For this review, take the finished solid that the model builds, in its own axes (mm). Round coordinates to 2 decimals unless told otherwise and drop trailing zeros. Write each loop counter-clockwise with the first axis right and the second up, starting at its lowest first coordinate (ties: lowest second). Pieces come first, ordered by that corner, then holes. Notation, with made-up numbers: (-4.75, -26.5) - (47.25, -26.5) arc R16 cw to (47.25, -1.5) - close; hole circle Ø5 at (54.25, 60.25). An arc over 180 degrees is marked (long way). One line per item, written item: value. Start each with the question number.
Q1. Add section B-B on y = 52. Write out the cut boundary in (x, z), and give its area (3 significant figures).
Q2. Clearance check with flat-ended pins moving along their axes: pin 1 Ø1 at (x, z) = (49, 2) entering from +Y; pin 2 Ø1.5 at (y, z) = (83, 1.5) entering from +X; pin 3 Ø11 at (x, y) = (0, 0) entering from +Z. State where each tip first meets the part, or that it passes through.
Q3. Add section A-A on z = 3.4. Write out the cut boundary in (x, y) (1 decimal).
Q4. Mouldability with a two-part tool opening along Y and no side actions: class faces 1 (the face through (-3.78, -2.9, 2.25)), 2 (the face through (63, -12.7, 2)), 3 (the face through (0, 68, 2)), 4 (the face through (70, 0, 2)) as +Y half, -Y half, draft (parallel to the pull), parting line (faces both ways), or undercut.
Q5. For probe 1 along X at (y, z) = (45, 2.35); probe 2 along Y at (x, z) = (-5, 1.8), list the stretches that pass through material, from the lowest coordinate up.
```python
from build123d import *

# Parameters (mm, degrees)
F0_R     = 4.7625
F1_DEPTH = 4.572
F2_R     = 2.032


with BuildPart() as f1:
    # F0 (on Top) → F1 (new body)
    with BuildSketch(Plane.XY):
        with BuildLine():
            ThreePointArc((0, -12.7), (8.980256, -8.980256), (12.7, 0))
            ThreePointArc((12.7, 0), (8.980256, 8.980256), (0, 12.7))
            ThreePointArc((0, 12.7), (-8.980256, 8.980256), (-12.7, 0))
            ThreePointArc((-12.7, 0), (-8.980256, -8.980256), (0, -12.7))
        make_face()
        Circle(F0_R, mode=Mode.SUBTRACT)
        with BuildLine():
            Line((127, 0), (12.7, 0))
            ThreePointArc((12.7, 0), (8.980256, -8.980256), (0, -12.7))
            Line((0, -12.7), (127, -12.7))
            Line((127, -12.7), (127, 0))
        make_face()
        with BuildLine():
            ThreePointArc((-12.7, 0), (-8.980256, 8.980256), (0, 12.7))
            Line((0, 12.7), (0, 126.691781))
            Line((0, 126.691781), (-12.7, 126.691781))
            Line((-12.7, 126.691781), (-12.7, 0))
        make_face()
    extrude(amount=F1_DEPTH)

    # F2
    f2_edges = [f1.edges().sort_by_distance(p)[0] for p in [
        (0, 126.691781, 2.286),
        (127, 0, 2.286),
    ]]
    fillet(f2_edges, radius=F2_R)


solid = f1.part
```
Result set:
1. outline: (-12.7, 0) - (0, 0) - (0, 4.57) - (-12.7, 4.57) - close
1. area: 58.1 mm^2
2. pin 1: stops at y = 0
2. pin 2: stops at x = 0
2. pin 3: stops at z = 4.57
3. outline: (-12.7, 0) arc R12.7 ccw to (0, -12.7) - (127, -12.7) - (127, -2) arc R2 ccw to (125, 0) - (12.7, 0) arc R12.7 ccw to (0, 12.7) - (0, 124.7) arc R2 ccw to (-2, 126.7) - (-12.7, 126.7) - close; hole circle Ø9.5 at (0, 0)
4. face 1: undercut
4. face 2: -Y half
4. face 3: draft
4. face 4: +Y half
5. probe 1: x = -12.7 to 0
5. probe 2: y = -11.67 to 126.69
